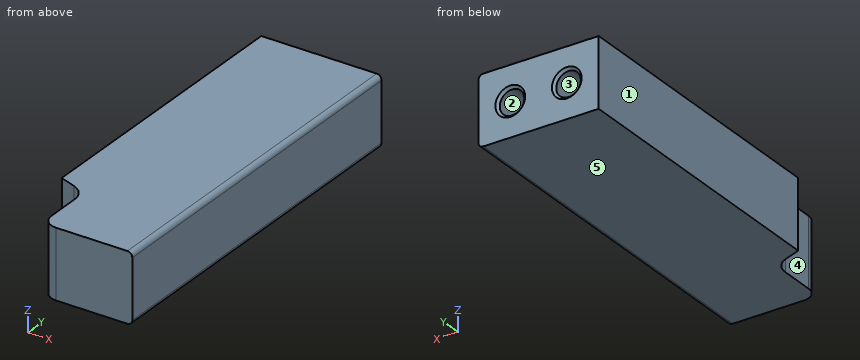
from build123d import *

# Parameters (mm, degrees)
SKETCH1_W                   = 24.5
SKETCH1_H                   = 14
BOSS_EXTRUDE1_DEPTH         = 75
CUT_EXTRUDE1_REACH          = 79.273
FILLET1_R                   = 3
FILLET2_R                   = 1
M6_TAPPED_HOLE1_D           = 5
M6_TAPPED_HOLE1_DEPTH       = 17
M6_TAPPED_HOLE1_CSINK_D     = 6.05
M6_TAPPED_HOLE1_CSINK_ANGLE = 90
M6_TAPPED_HOLE1_TIP         = 1.502151548


with BuildPart() as part:
    # Sketch1 → Boss-Extrude1 (new body)
    with BuildSketch(Plane(origin=(0, 0, 0), x_dir=(1, 0, 0), z_dir=(0, 1, 0))):
        Rectangle(SKETCH1_W, SKETCH1_H)
    extrude(amount=-BOSS_EXTRUDE1_DEPTH)

    # Sketch2 → Cut-Extrude1 (cut, up to next)
    with BuildSketch(Plane.XY.offset(7), mode=Mode.PRIVATE) as cut_extrude1_sk1:
        with BuildLine():
            Line((-8.881919427, -61.241229517), (-12.25, -60.015348442))
            Line((-12.25, -60.015348442), (-12.25, -75))
            Line((-12.25, -75), (-6.25, -75))
            Line((-6.25, -75), (-6.25, -65))
            ThreePointArc((-6.25, -65), (-6.973391823, -62.705694255), (-8.881919427, -61.241229517))
        make_face()
    cut_extrude1_tool1 = extrude(cut_extrude1_sk1.sketch, amount=-CUT_EXTRUDE1_REACH, mode=Mode.PRIVATE) & part.part
    add(cut_extrude1_tool1.solids().sort_by_distance((-9.372504, -68.134359, 7))[0], mode=Mode.SUBTRACT)

    # Fillet1
    fillet1_edges = [part.edges().sort_by_distance(p)[0] for p in [
        (-6.25, -75, 0),
    ]]
    fillet(fillet1_edges, radius=FILLET1_R)

    # Fillet2
    fillet2_edges = [part.edges().sort_by_distance(p)[0] for p in [
        (12.25, -37.5, 7),
        (12.25, -37.5, -7),
    ]]
    fillet(fillet2_edges, radius=FILLET2_R)

    # M6 Tapped Hole1
    with Locations(Plane(origin=(0, 0, 0), x_dir=(1, 0, 0), z_dir=(0, 1, 0))):
        with Locations((-5.75, 0), (5.75, 0)):
            CounterSinkHole(M6_TAPPED_HOLE1_D / 2, M6_TAPPED_HOLE1_CSINK_D / 2, depth=M6_TAPPED_HOLE1_DEPTH, counter_sink_angle=M6_TAPPED_HOLE1_CSINK_ANGLE)
            with Locations((0, 0, -(M6_TAPPED_HOLE1_DEPTH + M6_TAPPED_HOLE1_TIP / 2))):  # 118° drill point
                Cone(0, M6_TAPPED_HOLE1_D / 2, M6_TAPPED_HOLE1_TIP, mode=Mode.SUBTRACT)


solid = part.part
Verification items for the finished model (mm, model axes). Face numbers are marked on the shaded views. A direction names the side the tool comes from. Give positions to 0.01 mm unless a question says otherwise; leave off trailing zeros. Loops run counter-clockwise (first coordinate to the right, second up) from the corner with the lowest first, then second, coordinate; pieces in that order, holes last.
1. Go/stop test with flat-tipped pins: P1, Ø2, axis at y = -69, z = -2, coming from the -X side; P2, Ø4.5, axis at x = -5.75, z = 0, coming from the -Y side. Record where each tip stops, or that it passes through.
Derived:
P1: stops at x = -6.25
P2: stops at y = -74.99
2. Material ranges on probe 1 along Z at (x, y) = (-5.75, -5); probe 2 along Z at (x, y) = (-7.5, -7.5); probe 3 along X at (y, z) = (-63, -1.5), recorded low to high.
Derived:
probe 1: z = -7 to -2.5, 2.5 to 7
probe 2: z = -7 to -1.79, 1.79 to 7
probe 3: x = -6.79 to 12.25
3. Cross-section at A-A on z = 5. Record the cut outline in (x, y).
Derived:
outline: (-12.25, -60.02) - (-8.88, -61.24) arc R4 cw to (-6.25, -65) - (-6.25, -72) arc R3 ccw to (-3.25, -75) - (12.25, -75) - (12.25, 0) - (-12.25, 0) - close
4. Tool access check on the marked faces 1 and 2. Record the directions out of +Z, -Z, +X, -X, +Y, -Y that give a thin tool (end or side, any length) a straight path to the whole face; none if there is none.
Derived:
face 1: +Z, -Z, -X, +Y, -Y
face 2: +Y
5. Release check for a two-part mould opening along X. For the marked faces 3, 4 and 5 record: +X half, -X half, draft (parallel to the pull), parting line (faces both ways), or undercut.
Derived:
face 3: undercut
face 4: -X half
face 5: draft
